For this review, take the finished solid that the model builds, in its own axes (mm). A direction names the side the tool comes from. Coordinates: 2 decimals unless noted, no trailing zeros. Loops run counter-clockwise (first coordinate to the right, second up) from the corner with the lowest first, then second, coordinate; pieces in that order, holes last. Notation, with made-up numbers: M 38.25,44 L 74.25,44 A20 ccw 74.25,72 Z; hole C 28.5,-11 d9. An arc over 180 degrees is marked long. Put each result on its own line as item: value.
```python
from build123d import *

# Parameters (mm, degrees)
EXTRUDE_1_DEPTH = 1
FILLET_1_R      = 1
SKETCH_2_W      = 6
SKETCH_2_H      = 8
EXTRUDE_2_DEPTH = 3


with BuildPart() as part:
    # Эскиз1 → Бобышка-Вытянуть1 (new body)
    with BuildSketch(Plane.XY):
        Polygon((23, -22), (23, -26), (32.5, -26), (32.5, 26), (23, 26), (23, 22), (15, 22.030768978), (15, 26), (-32.5, 26), (-32.5, -26), (15, -26), (15, -22.030768978), align=None)
        with BuildLine():
            ThreePointArc((-20.75, 20), (-18.5, 22.25), (-20.75, 24.5))
            Line((-20.75, 24.5), (-23.75, 24.5))
            ThreePointArc((-23.75, 24.5), (-26, 22.25), (-23.75, 20))
            Line((-23.75, 20), (-20.75, 20))
        make_face(mode=Mode.SUBTRACT)
        with BuildLine():
            Line((-23.75, -20), (-20.75, -20))
            ThreePointArc((-20.75, -20), (-18.5, -22.25), (-20.75, -24.5))
            Line((-20.75, -24.5), (-23.75, -24.5))
            ThreePointArc((-23.75, -24.5), (-26, -22.25), (-23.75, -20))
        make_face(mode=Mode.SUBTRACT)
    extrude(amount=EXTRUDE_1_DEPTH)

    # Скругление1
    fillet_1_edges = [part.edges().sort_by_distance(p)[0] for p in [
        (23, -22, 0.5),
        (15, -22.030768978, 0.5),
        (15, -26, 0.5),
        (-32.5, -26, 0.5),
        (-32.5, 26, 0.5),
        (15, 26, 0.5),
        (15, 22.030768978, 0.5),
        (23, 22, 0.5),
        (23, 26, 0.5),
        (32.5, 26, 0.5),
        (32.5, -26, 0.5),
        (23, -26, 0.5),
    ]]
    fillet(fillet_1_edges, radius=FILLET_1_R)

    # Эскиз2 → Бобышка-Вытянуть2 (add)
    with BuildSketch(Plane.XY.offset(1)):
        with Locations((-30.5, 0)):
            Rectangle(SKETCH_2_W, SKETCH_2_H)
    extrude(amount=EXTRUDE_2_DEPTH)


solid = part.part
```
(1) Add section A-A (z = 2.3). Write out the cut boundary in (x, y).
Determined:
outline: M -33.5,-4 L -27.5,-4 L -27.5,4 L -33.5,4 Z
(2) Wall thickness on line 1 along Y through (x, z) = (-23, 0.6); line 2 along X through (y, z) = (-3.5, 3.05); line 3 along Z through (x, y) = (29.5, 15): over which ranges is each line inside the solid? List them lowest first. Write a range as [from, to].
Determined:
line 1: y = [-26, -24.5], [-20, 20], [24.5, 26]
line 2: x = [-33.5, -27.5]
line 3: z = [0, 1]
(3) Add section B-B (y = -13). Write out the cut boundary in (x, z).
Determined:
outline: M -32.5,0 L 32.5,0 L 32.5,1 L -32.5,1 Z
(4) Draft analysis for pull direction X (two halves, no side actions). For faces 5 (the flat face through (-31, 4, 2)), 6 (the flat face through (-33.5, 0, 2)), 7 (the cylindrical face through (-18.5, -22.2, 0.5)), state which applies: +X half, -X half, draft (parallel to the pull), parting line (faces both ways), or undercut.
Determined:
face 5: draft
face 6: -X half
face 7: undercut
(5) For pin 1 (4 mm diameter, centred on x = -20, y = -19, fed in from +Z); pin 2 (0.8 mm diameter, centred on y = -23.5, z = 0.5, fed in from -X); pin 3 (0.5 mm diameter, centred on x = -33, y = 1.5, fed in from -Z); pin 4 (4 mm diameter, centred on x = 2.5, y = 10, fed in from -Z), all flat-tipped, find the tip position at first contact; note any pin that passes through.
Determined:
pin 1: stops at z = 1
pin 2: stops at x = -32.5
pin 3: stops at z = 1
pin 4: stops at z = 0
(6) Tool access review of faces 1 (the flat face through (-27.5, 0, 2)), 2 (the cylindrical face through (-26, -22.3, 0.5)), 3 (the flat face through (-31, -4, 2)), 4 (the flat face through (0, 0, 0)): name each direction out of +Z, -Z, +X, -X, +Y, -Y from which nothing blocks a thin tool from reaching the whole face with its end or side.
Determined:
face 1: +Z, +X, +Y, -Y
face 2: +Z, -Z
face 3: +Z, +X, -X, -Y
face 4: -Z, +X, -X, +Y, -Y
